```python
from build123d import *

# Parameters (mm, degrees)
SKETCH_2_W          = 42.5
SKETCH_2_H          = 26
EXTRUDE_1_DEPTH     = 2.3
EXTRUDE_3_DEPTH     = 2.3
SKETCH_5_W          = 9
SKETCH_5_H          = 2.3
EXTRUDE_6_DEPTH     = 25
FILLET_1_R          = 2
CUT_EXTRUDE_1_REACH = 47.973
SKETCH_6_R          = 1.75
CUT_EXTRUDE_2_REACH = 49.209
SKETCH_7_R          = 1.25


with BuildPart() as part:
    # Sketch 2 → Extrude 1 (new body)
    with BuildSketch(Plane(origin=(0, 0, 0), x_dir=(1, 0, 0), z_dir=(0, 1, 0))):
        Rectangle(SKETCH_2_W, SKETCH_2_H)
    extrude(amount=EXTRUDE_1_DEPTH)

    # Sketch 3 → Extrude 3 (add)
    with BuildSketch(Plane(origin=(0, 0, -13), x_dir=(-1, 0, 0), z_dir=(0, 0, -1))):
        Polygon((20.25, 33), (20.25, 26.981475126), (18.25, 26.981475126), (18.25, 37), (-18.25, 37), (-18.25, 26.981475126), (-20.25, 26.981475126), (-20.25, 33), (-29.25, 33), (-29.25, 8.5), (-21.25, 8.5), (-21.25, 0), (21.25, 0), (21.25, 8.5), (29.25, 8.5), (29.25, 33), align=None)
    extrude(amount=-EXTRUDE_3_DEPTH)

    # Sketch 5 → Extrude 6 (add)
    with BuildSketch(Plane(origin=(0, 0, -13), x_dir=(-1, 0, 0), z_dir=(0, 0, -1))):
        with Locations((-24.75, 31.85)):
            Rectangle(SKETCH_5_W, SKETCH_5_H)
        with Locations((24.75, 31.85)):
            Rectangle(SKETCH_5_W, SKETCH_5_H)
    extrude(amount=-EXTRUDE_6_DEPTH)

    # Fillet 1
    fillet_1_edges = [part.edges().sort_by_distance(p)[0] for p in [
        (29.25, 8.5, -11.85),
        (18.25, 37, -11.85),
        (-18.25, 37, -11.85),
        (-29.25, 8.5, -11.85),
        (-24.75, 33, -13),
        (24.75, 33, -13),
        (0, 0, -13),
        (29.25, 31.85, 12),
        (20.25, 31.85, 12),
        (21.25, 1.15, 13),
        (-21.25, 1.15, 13),
        (-20.25, 31.85, 12),
        (-29.25, 31.85, 12),
    ]]
    fillet(fillet_1_edges, radius=FILLET_1_R)

    # Sketch 6 → Cut-Extrude 1 (cut, up to next)
    with BuildSketch(Plane(origin=(0, 33, 0), x_dir=(1, 0, 0), z_dir=(0, 1, 0)), mode=Mode.PRIVATE) as cut_extrude_1_sk1:
        with Locations(Location((-25, -5.75, 0), (0, 0, 270))):
            Circle(SKETCH_6_R)
    cut_extrude_1_tool1 = extrude(cut_extrude_1_sk1.sketch, amount=-CUT_EXTRUDE_1_REACH, mode=Mode.PRIVATE) & part.part
    # Sketch 6 → Cut-Extrude 1 (cut, up to next)
    with BuildSketch(Plane(origin=(0, 33, 0), x_dir=(1, 0, 0), z_dir=(0, 1, 0)), mode=Mode.PRIVATE) as cut_extrude_1_sk2:
        with Locations(Location((-25, 4.25, 0), (0, 0, 270))):
            Circle(SKETCH_6_R)
    cut_extrude_1_tool2 = extrude(cut_extrude_1_sk2.sketch, amount=-CUT_EXTRUDE_1_REACH, mode=Mode.PRIVATE) & part.part
    cut_extrude_1_1 = cut_extrude_1_tool1.solids().sort_by_distance((-25, 33, 5.75))[0]
    add(cut_extrude_1_1, mode=Mode.SUBTRACT)
    cut_extrude_1_2 = cut_extrude_1_tool2.solids().sort_by_distance((-25, 33, -4.25))[0]
    add(cut_extrude_1_2, mode=Mode.SUBTRACT)
    cut_extrude_1 = cut_extrude_1_1 + cut_extrude_1_2  # Cut-Extrude 1 as one shape, for the pattern or mirror that repeats it

    # Sketch 7 → Cut-Extrude 2 (cut, up to next)
    with BuildSketch(Plane(origin=(0, 2.3, 0), x_dir=(1, 0, 0), z_dir=(0, 1, 0)), mode=Mode.PRIVATE) as cut_extrude_2_sk1:
        with Locations(Location((-10.25, -0.75, 0), (0, 0, 270))):
            Circle(SKETCH_7_R)
    cut_extrude_2_tool1 = extrude(cut_extrude_2_sk1.sketch, amount=-CUT_EXTRUDE_2_REACH, mode=Mode.PRIVATE) & part.part
    # Sketch 7 → Cut-Extrude 2 (cut, up to next)
    with BuildSketch(Plane(origin=(0, 2.3, 0), x_dir=(1, 0, 0), z_dir=(0, 1, 0)), mode=Mode.PRIVATE) as cut_extrude_2_sk2:
        with Locations(Location((-10.25, -7.85, 0), (0, 0, 270))):
            Circle(SKETCH_7_R)
    cut_extrude_2_tool2 = extrude(cut_extrude_2_sk2.sketch, amount=-CUT_EXTRUDE_2_REACH, mode=Mode.PRIVATE) & part.part
    # Sketch 7 → Cut-Extrude 2 (cut, up to next)
    with BuildSketch(Plane(origin=(0, 2.3, 0), x_dir=(1, 0, 0), z_dir=(0, 1, 0)), mode=Mode.PRIVATE) as cut_extrude_2_sk3:
        with Locations(Location((-17.35, -0.75, 0), (0, 0, 270))):
            Circle(SKETCH_7_R)
    cut_extrude_2_tool3 = extrude(cut_extrude_2_sk3.sketch, amount=-CUT_EXTRUDE_2_REACH, mode=Mode.PRIVATE) & part.part
    # Sketch 7 → Cut-Extrude 2 (cut, up to next)
    with BuildSketch(Plane(origin=(0, 2.3, 0), x_dir=(1, 0, 0), z_dir=(0, 1, 0)), mode=Mode.PRIVATE) as cut_extrude_2_sk4:
        with Locations(Location((-10.25, 6.35, 0), (0, 0, 270))):
            Circle(SKETCH_7_R)
    cut_extrude_2_tool4 = extrude(cut_extrude_2_sk4.sketch, amount=-CUT_EXTRUDE_2_REACH, mode=Mode.PRIVATE) & part.part
    # Sketch 7 → Cut-Extrude 2 (cut, up to next)
    with BuildSketch(Plane(origin=(0, 2.3, 0), x_dir=(1, 0, 0), z_dir=(0, 1, 0)), mode=Mode.PRIVATE) as cut_extrude_2_sk5:
        with Locations(Location((-3.15, -0.75, 0), (0, 0, 270))):
            Circle(SKETCH_7_R)
    cut_extrude_2_tool5 = extrude(cut_extrude_2_sk5.sketch, amount=-CUT_EXTRUDE_2_REACH, mode=Mode.PRIVATE) & part.part
    cut_extrude_2_1 = cut_extrude_2_tool1.solids().sort_by_distance((-10.25, 2.3, 0.75))[0]
    add(cut_extrude_2_1, mode=Mode.SUBTRACT)
    cut_extrude_2_2 = cut_extrude_2_tool2.solids().sort_by_distance((-10.25, 2.3, 7.85))[0]
    add(cut_extrude_2_2, mode=Mode.SUBTRACT)
    cut_extrude_2_3 = cut_extrude_2_tool3.solids().sort_by_distance((-17.35, 2.3, 0.75))[0]
    add(cut_extrude_2_3, mode=Mode.SUBTRACT)
    cut_extrude_2_4 = cut_extrude_2_tool4.solids().sort_by_distance((-10.25, 2.3, -6.35))[0]
    add(cut_extrude_2_4, mode=Mode.SUBTRACT)
    cut_extrude_2_5 = cut_extrude_2_tool5.solids().sort_by_distance((-3.15, 2.3, 0.75))[0]
    add(cut_extrude_2_5, mode=Mode.SUBTRACT)
    cut_extrude_2 = cut_extrude_2_1 + cut_extrude_2_2 + cut_extrude_2_3 + cut_extrude_2_4 + cut_extrude_2_5  # Cut-Extrude 2 as one shape, for the pattern or mirror that repeats it

    # Mirror 1: Cut-Extrude 1, Cut-Extrude 2 across plane
    add(cut_extrude_1.mirror(Plane(origin=(0, 0, 0), x_dir=(0, 0, 1), z_dir=(1, 0, 0))), mode=Mode.SUBTRACT)
    add(cut_extrude_2.mirror(Plane(origin=(0, 0, 0), x_dir=(0, 0, 1), z_dir=(1, 0, 0))), mode=Mode.SUBTRACT)


solid = part.part
```
The listing builds one solid part. Answer for the finished solid, in the listing's coordinates (mm). A direction names the side the tool comes from. Round coordinates to 2 decimals unless told otherwise and drop trailing zeros. Loops run counter-clockwise (first coordinate to the right, second up) from the corner with the lowest first, then second, coordinate; pieces in that order, holes last.
Q1. Given pin 1 Ø3 at (x, z) = (-3.15, 0.75) entering from +Y; pin 2 Ø7 at (y, z) = (4.5, -5) entering from -X; pin 3 Ø7 at (x, z) = (25, -2.5) entering from +Y; pin 4 Ø12 at (x, z) = (-3.5, 6) entering from -Y, each flat-ended and moving along its own axis, determine where each tip first touches the part or whether it passes through.
Q2. Find the intervals of material crossed by line 1 (X direction, y = 31.5, z = 5.75); line 2 (X direction, y = 1.05, z = -6.35); line 3 (Y direction, x = -19.5, z = 10.25), in increasing order.
Q3. Section A-A, the plane x = -3.15 is taken. Determine the outline of the cut face in (y, z).
Q4. Which of the six approach directions +Z, -Z, +X, -X, +Y, -Y give full straight-line access (tool end or side, diameter ignored) to faces 4 (the face through (18.25, 31, -12)), 5 (the face through (-20.85, 31.87, 11.43)), 6 (the face through (-24.69, 32.4, -12.43))?
Q5. For a pull along Z with two mould halves and no side action, classify faces 1 (the face through (-24, 8.5, -12)), 2 (the face through (20.65, 1.17, 12.43)), 3 (the face through (-4.37, 1.17, 0.48)) as released by +Z, released by -Z, zero draft, split by the parting line, or undercut.
Q6. Section B-B, the plane x = 10.25 is taken. Determine the outline of the cut face in (y, z).
Q7. Section C-C, the plane z = -1.25 is taken. Determine the outline of the cut face in (x, y), then the cut area to 3 significant figures.
Q8. Section D-D, the plane x = 25 is taken. Determine the outline of the cut face in (y, z).
Completed:
1. pin 1: stops at y = 2.3
1. pin 2: stops at x = -21.25
1. pin 3: stops at y = 33
1. pin 4: stops at y = 0
2. line 1: x = -29.25 to -26.75, -23.25 to -20.25, 20.25 to 23.25, 26.75 to 29.25
2. line 2: x = -21.25 to -11.5, -9 to 9, 11.5 to 21.25
2. line 3: y = 0 to 2.3
3. outline: (0, -11) arc R2 ccw to (2, -13) - (37, -13) - (37, -10.7) - (2.3, -10.7) - (2.3, -0.5) - (0, -0.5) - close; (0, 2) - (2.3, 2) - (2.3, 13) - (0, 13) - close
4. face 4: +Z, -Z, +Y
4. face 5: +Z, +Y
4. face 6: -Z, -X, +Y
5. face 1: zero draft
5. face 2: released by +Z
5. face 3: undercut
6. outline: (0, -11) arc R2 ccw to (2, -13) - (37, -13) - (37, -10.7) - (2.3, -10.7) - (2.3, -7.6) - (0, -7.6) - close; (0, -5.1) - (2.3, -5.1) - (2.3, -0.5) - (0, -0.5) - close; (0, 2) - (2.3, 2) - (2.3, 6.6) - (0, 6.6) - close; (0, 9.1) - (2.3, 9.1) - (2.3, 13) - (0, 13) - close
7. outline: (-29.25, 30.7) - (-20.25, 30.7) - (-20.25, 33) - (-29.25, 33) - close; (-21.25, 0) - (21.25, 0) - (21.25, 2.3) - (-21.25, 2.3) - close; (20.25, 30.7) - (29.25, 30.7) - (29.25, 33) - (20.25, 33) - close
7. area: 139 mm2
8. outline: (8.5, -13) - (31, -13) arc R2 ccw to (33, -11) - (33, -6) - (30.7, -6) - (30.7, -10.7) - (8.5, -10.7) - close; (30.7, -2.5) - (33, -2.5) - (33, 4) - (30.7, 4) - close; (30.7, 7.5) - (33, 7.5) - (33, 12) - (30.7, 12) - close
